Check sheet for the modelled part. Datum: model origin and axes. Units: mm. Give positions to 0.01 mm unless a question says otherwise; leave off trailing zeros. Order: outer loops, then holes, each group sorted by start corner. A loop starts at its lowest first (then second) coordinate and runs counter-clockwise, first axis right, second up.
from build123d import *


with BuildPart() as f3:
    # F0 (on Top) → F3 section 0
    with BuildSketch(Plane.XY, mode=Mode.PRIVATE) as f3_s0:
        Polygon((-56.804541, -117.955845), (56.804541, -117.955845), (127.638645, -29.132688), (102.358246, 81.627977), (0, 130.921111), (-102.358246, 81.627977), (-127.638645, -29.132688), align=None)
    loft([f3_s0.sketch, Vertex(0, 0, 100)])


solid = f3.part
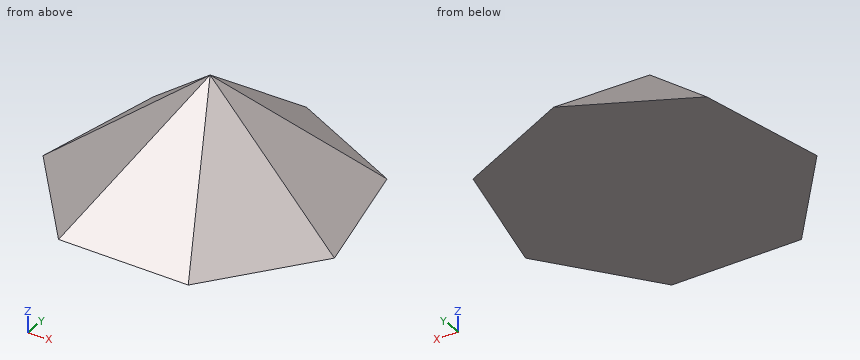
1) Section check A-A, the plane z = 21.5. Record the cut outline in (x, y).
Recorded:
outline: (-100.2, -22.87) - (-44.59, -92.6) - (44.59, -92.6) - (100.2, -22.87) - (80.35, 64.08) - (0, 102.77) - (-80.35, 64.08) - close
2) Section check D-D, the plane z = 80. Record the cut outline in (x, y).
Recorded:
outline: (-25.53, -5.83) - (-11.36, -23.59) - (11.36, -23.59) - (25.53, -5.83) - (20.47, 16.33) - (0, 26.18) - (-20.47, 16.33) - close
3) Section check C-C, the plane y = 12. Record the cut outline in (x, z).
Recorded:
outline: (-118.25, 0) - (118.25, 0) - (15.05, 85.3) - (0, 90.83) - (-15.05, 85.3) - close
4) Section check B-B, the plane x = 5.5. Record the cut outline in (y, z), then the cut area to 3 significant figures.
Recorded:
outline: (-117.96, 0) - (128.27, 0) - (4.39, 94.63) - (-1.26, 95.69) - (-11.42, 90.32) - close
area: 12,200 mm2
5) Depth check by flat-ended pin: pin 1 Ø12 at (y, z) = (30.5, 68) entering from +X; pin 2 Ø6 at (x, z) = (-3, 10.5) entering from +Y; pin 3 Ø2 at (y, z) = (-30, 66.5) entering from +X. Enter the tip coordinate at first touch or a pass-through.
Recorded:
pin 1: stops at x = 39.14
pin 2: stops at y = 119.91
pin 3: stops at x = 28.32
6) Material ranges on L1, parallel to Z at x = 78.5, y = -30.5; L2, parallel to Z at x = 97.5, y = 40; L3, parallel to Y at x = 12, z = 50.5, recorded low to high.
Recorded:
L1: z = 0 to 31.85
L2: z = 0 to 11.87
L3: y = -58.39 to 59.03
